Autodesk Inventor part; units mm, degrees
ref_plane "YZ Plane" through (0, 0, 0) normal (1, 0, 0) x (0, 1, 0)
ref_plane "XZ Plane" through (0, 0, 0) normal (0, 1, 0) x (-1, 0, 0)
ref_plane "XY Plane" through (0, 0, 0) normal (0, 0, 1) x (1, 0, 0)
sketch "Sketch1" plane through (0, 0, 0) normal (0, 0, 1) x (1, 0, 0)
  line L0 (0, 0) -> (25.908, 0)
  line L1 (25.908, 0) -> (25.908, 25.908)
  line L2 (25.908, 25.908) -> (0, 25.908)
  line L3 (0, 25.908) -> (0, 0)
  line L4 (-6.35, 0) -> (-6.35, -6.35)
  line L5 (-6.35, -6.35) -> (0, -6.35)
  line L6 (-6.35, -6.35) -> (31.75, -6.35)
  line L7 (31.75, -6.35) -> (31.75, 31.75)
  line L8 (31.75, 31.75) -> (-6.35, 31.75)
  line L9 (-6.35, 31.75) -> (-6.35, -6.35)
  dimension "d0" = 25.908
  dimension "d1" = 25.908
  dimension "d4" = 38.1
  dimension "d5" = 38.1
extrude "Extrusion1" add sketch "Sketch1" along normal blind 38.1
sketch "Sketch2" plane through (-6.35, 31.75, 0) normal (0, 1, 0) x (1, 0, 0)
  line L0 (0, -38.1) -> (38.1, -38.1)
  line L1 (38.1, 0) -> (38.1, -38.1)
  line L2 (38.1, 0) -> (0, 0)
  line L3 (0, 0) -> (0, -38.1)
  line L4 (0, -38.1) -> (0, -19.05)
  line L5 (0, 0) -> (0, -38.1)
  point P0 (6.35, 0)
sketch "Sketch3" plane through (-6.35, 31.75, 0) normal (0, 1, 0) x (1, 0, 0)
  line L0 (0, -38.1) -> (38.1, -38.1)
  line L1 (38.1, 0) -> (38.1, -38.1)
  line L2 (38.1, 0) -> (0, 0)
  line L3 (0, 0) -> (0, -38.1)
  point P0 (6.35, 0)
  point P1 (38.1, -19.05)
sketch "Sketch4" plane through (0, 0, 38.1) normal (0, 0, 1) x (1, 0, 0)
  line L0 (0, 0) -> (25.908, 0)
  line L1 (25.908, 0) -> (25.908, -3.175)
  line L2 (25.908, -3.175) -> (0, -3.175)
  line L3 (0, -3.175) -> (0, 0)
  line L4 (25.908, 0) -> (29.083, 0)
  line L5 (29.083, 0) -> (29.083, 25.908)
  line L6 (29.083, 25.908) -> (25.908, 25.908)
  line L7 (25.908, 25.908) -> (25.908, 0)
  line L8 (25.908, 25.908) -> (0, 25.908)
  line L9 (0, 25.908) -> (0, 29.083)
  line L10 (0, 29.083) -> (25.908, 29.083)
  line L11 (25.908, 29.083) -> (25.908, 25.908)
  line L12 (0, 0) -> (-3.175, 0)
  line L13 (-3.175, 0) -> (-3.175, 25.908)
  line L14 (-3.175, 25.908) -> (0, 25.908)
  line L15 (0, 25.908) -> (0, 0)
  dimension "d8" = 3.175
  dimension "d9" = 3.175
  dimension "d10" = 3.175
  dimension "d11" = 3.175
extrude "Extrusion2" cut sketch "Sketch4" against normal blind 38.1 contours L0 L1 L2 L3 | L12 L13 L14 L15 | L7 L6 L5 L4 | L9 L10 L11 L8
sketch "Sketch5" plane through (0, 29.083, 38.1) normal (0, -1, 0) x (1, 0, 0)
  line L0 (0, 0) -> (0, -38.1)
  line L1 (0, 0) -> (0, -19.05)
  line L2 (0, -19.05) -> (12.954, -19.05)
  line L3 (25.908, 0) -> (25.908, -38.1)
  line L4 (12.954, -19.05) -> (12.954, -15.9258)
  line L5 (12.954, -15.9258) -> (15.6596, -17.4879)
  line L6 (15.6596, -17.4879) -> (15.6596, -20.6121)
  line L7 (15.6596, -20.6121) -> (12.954, -22.1742)
  line L8 (12.954, -22.1742) -> (10.2484, -20.6121)
  line L9 (10.2484, -20.6121) -> (10.2484, -17.4879)
  line L10 (10.2484, -17.4879) -> (12.954, -15.9258)
  dimension "d14" = 19.05
  dimension "d22" = 3.1242
extrude "Extrusion3" add sketch "Sketch5" along normal blind 2.54
sketch "Sketch6" plane through (-3.175, 0, 38.1) normal (1, 0, 0) x (0, 0, -1)
  line L0 (38.1, 25.908) -> (38.1, 0)
  line L1 (38.1, 0) -> (38.1, 12.954)
  line L2 (38.1, 12.954) -> (19.05, 12.954)
  line L3 (19.05, 12.954) -> (22.1742, 12.954)
  line L4 (22.1742, 12.954) -> (20.6121, 10.2484)
  line L5 (20.6121, 10.2484) -> (17.4879, 10.2484)
  line L6 (17.4879, 10.2484) -> (15.9258, 12.954)
  line L7 (15.9258, 12.954) -> (17.4879, 15.6596)
  line L8 (17.4879, 15.6596) -> (20.6121, 15.6596)
  line L9 (20.6121, 15.6596) -> (22.1742, 12.954)
  dimension "d19" = 12.954
  dimension "d20" = 19.05
  dimension "d23" = 3.1242
extrude "Extrusion4" add sketch "Sketch6" along normal blind 2.54
sketch "Sketch7" plane through (0, -3.175, 38.1) normal (0, 1, 0) x (1, 0, 0)
  line L0 (0, 0) -> (0, 38.1)
  line L1 (0, 0) -> (0, 19.05)
  line L2 (0, 19.05) -> (12.954, 19.05)
  line L3 (12.954, 19.05) -> (12.954, 15.9258)
  line L4 (12.954, 15.9258) -> (10.2484, 17.4879)
  line L5 (10.2484, 17.4879) -> (10.2484, 20.6121)
  line L6 (10.2484, 20.6121) -> (12.954, 22.1742)
  line L7 (12.954, 22.1742) -> (15.6596, 20.6121)
  line L8 (15.6596, 20.6121) -> (15.6596, 17.4879)
  line L9 (15.6596, 17.4879) -> (12.954, 15.9258)
  dimension "d26" = 19.05
  dimension "d27" = 12.954
  dimension "d28" = 3.1242
extrude "Extrusion5" add sketch "Sketch7" along normal blind 2.54
sketch "Sketch8" plane through (29.083, 0, 38.1) normal (-1, 0, 0) x (0, 0, 1)
  line L0 (0, 0) -> (-19.05, 0)
  line L1 (-38.1, 0) -> (0, 0)
  line L2 (-19.05, 0) -> (-19.05, 12.954)
  line L3 (-19.05, 12.954) -> (-15.9258, 12.954)
  line L4 (-15.9258, 12.954) -> (-17.4879, 10.2484)
  line L5 (-17.4879, 10.2484) -> (-20.6121, 10.2484)
  line L6 (-20.6121, 10.2484) -> (-22.1742, 12.954)
  line L7 (-22.1742, 12.954) -> (-20.6121, 15.6596)
  line L8 (-20.6121, 15.6596) -> (-17.4879, 15.6596)
  line L9 (-17.4879, 15.6596) -> (-15.9258, 12.954)
  dimension "d31" = 19.05
  dimension "d32" = 12.954
  dimension "d33" = 3.1242
extrude "Extrusion6" add sketch "Sketch8" along normal blind 2.54
sketch "Sketch9" plane through (0, 0, 38.1) normal (0, 0, 1) x (1, 0, 0)
  line L0 (0, 25.908) -> (0, 29.083)
  line L1 (0, 29.083) -> (25.908, 29.083)
  line L2 (25.908, 29.083) -> (25.908, 25.908)
  line L3 (25.908, 25.908) -> (29.083, 25.908)
  line L4 (29.083, 25.908) -> (29.083, 0)
  line L5 (29.083, 0) -> (25.908, 0)
  line L6 (25.908, 0) -> (25.908, -3.175)
  line L7 (25.908, -3.175) -> (0, -3.175)
  line L8 (0, -3.175) -> (0, 0)
  line L9 (0, 0) -> (-3.175, 0)
  line L10 (-3.175, 0) -> (-3.175, 25.908)
  line L11 (-3.175, 25.908) -> (0, 25.908)
  line L12 (-6.35, -6.35) -> (-6.35, 31.75)
  line L13 (31.75, -6.35) -> (-6.35, -6.35)
  line L14 (31.75, 31.75) -> (31.75, -6.35)
  line L15 (-6.35, 31.75) -> (31.75, 31.75)
extrude "Extrusion7" cut sketch "Sketch9" against normal blind 6.35
extrude "Extrusion8" cut sketch "Sketch1" along normal blind 6.35
properties part number "freeholder"
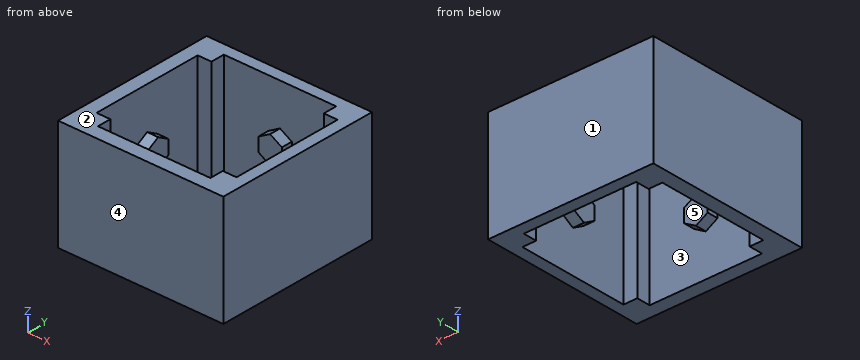
CAD build for the part. Positions are in the model's coordinates, mm. Face numbers are marked on the shaded views. A direction names the side the tool comes from. Give positions to 0.01 mm unless a question says otherwise; leave off trailing zeros. Order: outer loops, then holes, each group sorted by start corner. A loop starts at its lowest first (then second) coordinate and runs counter-clockwise, first axis right, second up. Notation, with made-up numbers: M 54.5,80 L 79.5,80 A13 cw 79.5,87 Z; hole C 25,16.5 d6. An arc over 180 degrees is marked long. Put each result on its own line as item: value. Start each with the question number.
(1) Saw through at C-C, the plane z = 15. Write the cut outline in (x, y) (3 decimals).
(2) Mould opens along Y. For the marked faces 1, 2 and 3 say: +Y half, -Y half, draft (parallel to the pull), parting line (faces both ways), or undercut.
(3) Saw through at A-A, the plane x = 16.5. Write the cut outline in (y, z) (3 decimals), then the cut area to 3 significant figures.
(4) Which spindle directions (+Z, -Z, +X, -X, +Y, -Y) get a long thin tool onto all of the face, cutting with end or side? Do the marked faces 4 and 5. Say none if no direction does.
(5) Drill centre lines: line 1 along X through (y, z) = (21, 24.5) (3 decimals); line 2 along X through (y, z) = (-0.5, 22.5). Where is each one in solid material? Low to high.
(6) Saw through at D-D, the plane y = 11.5. Write the cut outline in (x, z) (3 decimals), then the cut area to 3 significant figures.
Check result:
1. outline: M -6.35,-6.35 L 31.75,-6.35 L 31.75,31.75 L -6.35,31.75 Z; hole M -3.175,0 L 0,0 L 0,-3.175 L 25.908,-3.175 L 25.908,0 L 29.083,0 L 29.083,25.908 L 25.908,25.908 L 25.908,29.083 L 0,29.083 L 0,25.908 L -3.175,25.908 Z
2. face 1: +Y half
2. face 2: draft
2. face 3: undercut
3. outline: M -6.35,6.35 L -3.175,6.35 L -3.175,31.75 L -6.35,31.75 Z; M 29.083,6.35 L 31.75,6.35 L 31.75,31.75 L 29.083,31.75 Z
3. area: 148 mm2
4. face 4: +Z, -Z, +X, -X, -Y
4. face 5: +Z, -Z
5. line 1: x = -6.35 to -3.175, 29.083 to 31.75
5. line 2: x = -6.35 to 0, 25.91 to 31.75
6. outline: M -6.35,6.35 L -3.175,6.35 L -3.175,16.765 L -0.635,16.765 L -0.635,21.335 L -3.175,21.335 L -3.175,31.75 L -6.35,31.75 Z; M 26.543,16.765 L 29.083,16.765 L 29.083,6.35 L 31.75,6.35 L 31.75,31.75 L 29.083,31.75 L 29.083,21.335 L 26.543,21.335 Z
6. area: 172 mm2
